For this review, take the finished solid that the model builds, in its own axes (mm). A direction names the side the tool comes from. Coordinates: 2 decimals unless noted, no trailing zeros. Order: outer loops, then holes, each group sorted by start corner. A loop starts at its lowest first (then second) coordinate and runs counter-clockwise, first axis right, second up. Notation, with made-up numbers: (21, -27.75) -> (35, -27.75) arc R16 ccw to (35, -1.75) -> close; hole circle Ø9 at (-38, 59.5). An arc over 180 degrees is marked (long way). Answer as a JSON object with one key per item and string values. Group by question number.
1) Add section D-D, the plane x = 6.5. Write out the cut boundary in (y, z).
2) Draft analysis for pull direction Y (two halves, no side actions). For faces 1 (the flat face through (0, -20, 1)), 2 (the flat face through (0, 22.671, 4)), 3 (the flat face through (0, 50, 0)), 4 (the flat face through (0, 2, 6.5)), state which applies: +Y half, -Y half, draft (parallel to the pull), parting line (faces both ways), or undercut.
3) Add section C-C, the plane y = -13.5. Write out the cut boundary in (x, z), then the cut area to 4 significant figures.
4) For pin 1 (0.5 mm diameter, centred on x = -8.5, y = 23, fed in from +Z); pin 2 (10.5 mm diameter, centred on x = 18, y = -9, fed in from +Z); pin 3 (2.5 mm diameter, centred on x = 19.5, y = 11.5, fed in from -Z); pin 4 (1.2 mm diameter, centred on y = 3, z = 6, fed in from +X), all flat-tipped, find the tip position at first contact; note any pin that passes through.
5) Add section B-B, the plane y = 11.5. Write out the cut boundary in (x, z), then the cut area to 4 significant figures.
6) Add section A-A, the plane x = -19.5. Write out the cut boundary in (y, z), then the cut area to 3 significant figures.
7) Machinability: for faces 5 (the flat face through (0, 23.297, 4)), 6 (the flat face through (9.5, 1, 6)), 7 (the flat face through (0, 37, 5)), which of the approach directions +Z, -Z, +X, -X, +Y, -Y give a long, thin tool a straight path to every point of the face, cutting with its end or side? Answer none if there is none.
8) Wall thickness on L1, parallel to Y at x = 19.5, z = -1.25; L2, parallel to Z at x = 13.5, y = -2; L3, parallel to Y at x = -1, z = 3.75: over which ranges is each line inside the solid? List them lowest first.
from build123d import *

# Parameters (mm, degrees)
SKETCH2_W           = 45
SKETCH2_H           = 10
BOSS_EXTRUDE1_DEPTH = 40
SKETCH4_W           = 45
SKETCH4_H           = 10
BOSS_EXTRUDE2_DEPTH = 10
SKETCH8_W           = 45
SKETCH8_H           = 10
BOSS_EXTRUDE3_DEPTH = 20
SKETCH9_R           = 1.45
CUT_EXTRUDE2_DEPTH  = 20
SKETCH10_W          = 45
SKETCH10_H          = 0.626165357
CUT_EXTRUDE3_DEPTH  = 2
SKETCH11_W          = 19
SKETCH11_H          = 42.671327575
BOSS_EXTRUDE4_DEPTH = 1.5


with BuildPart() as part:
    # Sketch2 → Boss-Extrude1 (new body)
    with BuildSketch(Plane(origin=(0, 0, 0), x_dir=(1, 0, 0), z_dir=(0, 1, 0))):
        Rectangle(SKETCH2_W, SKETCH2_H)
    extrude(amount=BOSS_EXTRUDE1_DEPTH)

    # Sketch4 → Boss-Extrude2 (add)
    with BuildSketch(Plane(origin=(0, 40, 0), x_dir=(1, 0, 0), z_dir=(0, 1, 0))):
        Rectangle(SKETCH4_W, SKETCH4_H)
    extrude(amount=BOSS_EXTRUDE2_DEPTH)

    # Sketch8 → Boss-Extrude3 (add)
    with BuildSketch(Plane.XZ):
        Rectangle(SKETCH8_W, SKETCH8_H)
    extrude(amount=BOSS_EXTRUDE3_DEPTH)

    # Sketch9 → Cut-Extrude2 (cut)
    with BuildSketch(Plane.XY.offset(5)):
        with Locations((19.5, 11.5)):
            Circle(SKETCH9_R)
        with Locations((-19.5, 11.5)):
            Circle(SKETCH9_R)
    extrude(amount=-CUT_EXTRUDE2_DEPTH, mode=Mode.SUBTRACT)

    # Sketch10 → Cut-Extrude3 (cut)
    with BuildSketch(Plane.XY.offset(5)):
        with Locations((0, 22.984410254)):
            Rectangle(SKETCH10_W, SKETCH10_H)
    extrude(amount=-CUT_EXTRUDE3_DEPTH, mode=Mode.SUBTRACT)

    # Sketch11 → Boss-Extrude4 (add)
    with BuildSketch(Plane.XY.offset(5)):
        with Locations((0, 1.335663788)):
            Rectangle(SKETCH11_W, SKETCH11_H)
    extrude(amount=BOSS_EXTRUDE4_DEPTH)


solid = part.part
Output values:
{
 "1": {"outline": "(-20, -5) -> (50, -5) -> (50, 5) -> (23.3, 5) -> (23.3, 3) -> (22.67, 3) -> (22.67, 6.5) -> (-20, 6.5) -> close"},
 "2": {"face 1": "-Y half", "face 2": "undercut", "face 3": "+Y half", "face 4": "draft"},
 "3": {"outline": "(-22.5, -5) -> (22.5, -5) -> (22.5, 5) -> (9.5, 5) -> (9.5, 6.5) -> (-9.5, 6.5) -> (-9.5, 5) -> (-22.5, 5) -> close", "area": "478.5 mm²"},
 "4": {"pin 1": "stops at z = 3", "pin 2": "stops at z = 5", "pin 3": "passes through", "pin 4": "stops at x = 9.5"},
 "5": {"outline": "(-22.5, -5) -> (-20.95, -5) -> (-20.95, 5) -> (-22.5, 5) -> close; (-18.05, -5) -> (18.05, -5) -> (18.05, 5) -> (9.5, 5) -> (9.5, 6.5) -> (-9.5, 6.5) -> (-9.5, 5) -> (-18.05, 5) -> close; (20.95, -5) -> (22.5, -5) -> (22.5, 5) -> (20.95, 5) -> close", "area": "420.5 mm²"},
 "6": {"outline": "(-20, -5) -> (10.05, -5) -> (10.05, 5) -> (-20, 5) -> close; (12.95, -5) -> (50, -5) -> (50, 5) -> (23.3, 5) -> (23.3, 3) -> (22.67, 3) -> (22.67, 5) -> (12.95, 5) -> close", "area": "670 mm²"},
 "7": {"face 5": "+Z, +X, -X", "face 6": "+Z, +X, +Y, -Y", "face 7": "+Z, +X, -X, +Y"},
 "8": {"L1": "y = -20 to 10.05, 12.95 to 50", "L2": "z = -5 to 5", "L3": "y = -20 to 22.67, 23.3 to 50"}
}
